from build123d import *

# Parameters (mm, degrees)
IZIM1_W                     = 25
IZIM1_H                     = 34
Y_KSEKLIK_EKSTR_ZYON1_DEPTH = 7.04
IZIM2_W                     = 21
IZIM2_H                     = 30
IZIM2_R                     = 1.4
KES_EKSTR_ZYON1_DEPTH       = 5.04
IZIM3_W                     = 20
IZIM3_H                     = 5.688553579
KES_EKSTR_ZYON2_DEPTH       = 3.9
IZIM4_W                     = 2.2
IZIM4_H                     = 1.1
Y_KSEKLIK_EKSTR_ZYON2_DEPTH = 1.1
IZIM5_W                     = 1
IZIM5_H                     = 0.5
KES_EKSTR_ZYON3_DEPTH       = 2


with BuildPart() as part:
    # Çizim1 → Yükseklik-Ekstrüzyon1 (new body)
    with BuildSketch(Plane(origin=(0, 0, 0), x_dir=(1, 0, 0), z_dir=(0, 1, 0))):
        Rectangle(IZIM1_W, IZIM1_H)
    extrude(amount=Y_KSEKLIK_EKSTR_ZYON1_DEPTH)

    # Çizim2 → Kes-Ekstrüzyon1 (cut)
    with BuildSketch(Plane(origin=(0, 7.04, 0), x_dir=(1, 0, 0), z_dir=(0, 1, 0))):
        Rectangle(IZIM2_W, IZIM2_H)
        with Locations((-7, 11.5)):
            Circle(IZIM2_R, mode=Mode.SUBTRACT)
        with Locations((7, 11.5)):
            Circle(IZIM2_R, mode=Mode.SUBTRACT)
    extrude(amount=-KES_EKSTR_ZYON1_DEPTH, mode=Mode.SUBTRACT)

    # Çizim3 → Kes-Ekstrüzyon2 (cut)
    with BuildSketch(Plane(origin=(0, 7.04, 0), x_dir=(1, 0, 0), z_dir=(0, 1, 0))):
        with Locations((0, -14.80753211)):
            Rectangle(IZIM3_W, IZIM3_H)
    extrude(amount=-KES_EKSTR_ZYON2_DEPTH, mode=Mode.SUBTRACT)

    # Çizim4 → Yükseklik-Ekstrüzyon2 (add)
    with BuildSketch(Plane(origin=(0, 2, 0), x_dir=(1, 0, 0), z_dir=(0, 1, 0))):
        with Locations((0, 14.45)):
            Rectangle(IZIM4_W, IZIM4_H)
    extrude(amount=Y_KSEKLIK_EKSTR_ZYON2_DEPTH)

    # Çizim5 → Kes-Ekstrüzyon3 (cut)
    with BuildSketch(Plane(origin=(0, 7.04, 0), x_dir=(1, 0, 0), z_dir=(0, 1, 0))):
        with Locations((-10, -16)):
            Rectangle(IZIM5_W, IZIM5_H)
        with Locations((10, -16)):
            Rectangle(IZIM5_W, IZIM5_H)
    extrude(amount=-KES_EKSTR_ZYON3_DEPTH, mode=Mode.SUBTRACT)


solid = part.part
CAD build for the part. Positions are in the model's coordinates, mm. A direction names the side the tool comes from. Give positions to 0.01 mm unless a question says otherwise; leave off trailing zeros. Loops run counter-clockwise (first coordinate to the right, second up) from the corner with the lowest first, then second, coordinate; pieces in that order, holes last. Notation, with made-up numbers: M 81.25,29.5 L 118.25,29.5 A15 cw 118.25,48.5 Z; hole C 76,-22.5 d10. An arc over 180 degrees is marked long. Answer in a Markdown table with one row per item. Add a question column.
Item 1: Band-saw the part on D-D on z = 2.5. Give the cut face in (x, y), then the cut area to 3 significant figures.
Item 2: Band-saw the part on B-B on x = -3.25. Give the cut face in (y, z).
Item 3: Drop flat-ended pins along their axis: P1, Ø1, axis at x = 5, z = 13, coming from the -Y side; P2, Ø1.6, axis at x = 0, z = 16, coming from the +Y side; P3, Ø10.5, axis at x = -1.5, z = 1, coming from the +Y side. Give the stop position or say it passes through.
Item 4: Probe probe 1 along X at (y, z) = (4.5, -14.5); probe 2 along Z at (x, y) = (-10, 2.5); probe 3 along Z at (x, y) = (-8, 3). List the from-to ranges inside material, lowest first.
Item 5: Band-saw the part on C-C on z = -11.5. Give the cut face in (x, y), then the cut area to 3 significant figures.
Item 6: Mould opens along Z. For faces 1 (the face through (0, 2, 17)), 2 (the face through (-10, 4.7, 16)), 3 (the face through (0, 3, -17)), 4 (the face through (-10.5, 5, 0)) say: +Z half, -Z half, draft (parallel to the pull), parting line (faces both ways), or undercut.
Item 7: Band-saw the part on A-A on y = 5.5. Give the cut face in (x, z), then the cut area to 3 significant figures.
Item 8: Tool access for faces 5 (the face through (12.5, 3, 0)), 6 (the face through (6.82, 4.56, -12.89)), 7 (the face through (10, 4.7, 16)): list every direction of +Z, -Z, +X, -X, +Y, -Y with a clear straight run to the whole face (end or side of a thin tool).
Reply:
| question | item | result |
|---|---|---|
| 1 | outline | M -12.5,0 L 12.5,0 L 12.5,7.04 L 10.5,7.04 L 10.5,2 L -10.5,2 L -10.5,7.04 L -12.5,7.04 Z |
| 1 | area | 70.2 mm^2 |
| 2 | outline | M 0,-17 L 7.04,-17 L 7.04,-15 L 2,-15 L 2,15 L 3.14,15 L 3.14,17 L 0,17 Z |
| 3 | P1 | stops at y = 0 |
| 3 | P2 | stops at y = 3.14 |
| 3 | P3 | stops at y = 2 |
| 4 | probe 1 | x = -12.5 to -10.5, 10.5 to 12.5 |
| 4 | probe 2 | z = -17 to -15, 15 to 17 |
| 4 | probe 3 | z = -17 to -15, -12.48 to -10.52, 15 to 17 |
| 5 | outline | M -12.5,0 L 12.5,0 L 12.5,7.04 L 10.5,7.04 L 10.5,2 L 8.4,2 L 8.4,7.04 L 5.6,7.04 L 5.6,2 L -5.6,2 L -5.6,7.04 L -8.4,7.04 L -8.4,2 L -10.5,2 L -10.5,7.04 L -12.5,7.04 Z |
| 5 | area | 98.4 mm^2 |
| 6 | face 1 | +Z half |
| 6 | face 2 | draft |
| 6 | face 3 | -Z half |
| 6 | face 4 | undercut |
| 7 | outline | M -12.5,-17 L 12.5,-17 L 12.5,17 L 10,17 L 10,16.25 L 10.5,16.25 L 10.5,15.75 L 10,15.75 L 10,15 L 10.5,15 L 10.5,-15 L -10.5,-15 L -10.5,15 L -10,15 L -10,15.75 L -10.5,15.75 L -10.5,16.25 L -10,16.25 L -10,17 L -12.5,17 Z; C -7,-11.5 d2.8; C 7,-11.5 d2.8 |
| 7 | area | 192 mm^2 |
| 8 | face 5 | +Z, -Z, +X, +Y, -Y |
| 8 | face 6 | +Y |
| 8 | face 7 | +Z, +Y |
